Read the model definition and answer for the solid it produces. Units are mm, in the model's axes. Face numbers are marked on the shaded views. Coordinates: 2 decimals unless noted, no trailing zeros. Write each loop counter-clockwise with the first axis right and the second up, starting at its lowest first coordinate (ties: lowest second). Pieces come first, ordered by that corner, then holes. Notation, with made-up numbers: (66, -24) - (122, -24) arc R32 ccw to (122, 10) - close; hole circle Ø4 at (-12.75, 73.25). An arc over 180 degrees is marked (long way). Return JSON: item names as keys, results as strings.
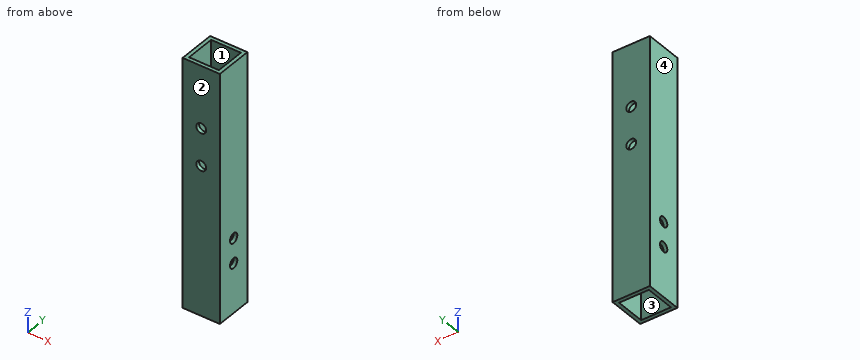
```python
from build123d import *

# Parameters (mm, degrees)
SKETCH_1_W          = 15
SKETCH_1_H          = 15
SKETCH_1_W_2        = 12
SKETCH_1_H_2        = 12
EXTRUDE_1_DEPTH     = 100
SKETCH_4_R          = 2
CUT_EXTRUDE_2_DEPTH = 75
SKETCH_5_R          = 2
CUT_EXTRUDE_3_DEPTH = 102.396498953


with BuildPart() as part:
    # 草图1 → 凸台-拉伸1 (new body)
    with BuildSketch(Plane.XY):
        Rectangle(SKETCH_1_W, SKETCH_1_H)
        Rectangle(SKETCH_1_W_2, SKETCH_1_H_2, mode=Mode.SUBTRACT)
    extrude(amount=EXTRUDE_1_DEPTH)

    # 草图4 → 切除-拉伸2 (cut)
    with BuildSketch(Plane.XZ.offset(7.5)):
        with Locations(Location((0, 75, 0), (0, 0, 270))):
            Circle(SKETCH_4_R)
        with Locations(Location((0, 60, 0), (0, 0, 270))):
            Circle(SKETCH_4_R)
    extrude(amount=-CUT_EXTRUDE_2_DEPTH, mode=Mode.SUBTRACT)

    # 草图5 → 切除-拉伸3 (cut, through all)
    with BuildSketch(Plane.ZY.offset(7.5)):
        with Locations((20, 0)):
            Circle(SKETCH_5_R)
        with Locations((30, 0)):
            Circle(SKETCH_5_R)
    extrude(amount=-CUT_EXTRUDE_3_DEPTH, mode=Mode.SUBTRACT)


solid = part.part
```
(1) A cutting plane is placed at D-D (x = -3.75). Determine the outline of the cut face in (y, z), and give its area (3 significant figures).
Answer:
{"outline": "(-7.5, 0) - (-6, 0) - (-6, 100) - (-7.5, 100) - close; (6, 0) - (7.5, 0) - (7.5, 100) - (6, 100) - close", "area": "300 mm²"}
(2) Straight lines are drawn through the part: line 1 (Y direction, x = 1, z = 38); line 2 (X direction, y = 7.15, z = 75). For each, find the intervals that lie inside material, in ascending order. Write a range as from..to.
Answer:
{"line 1": "-7.5..-6, 6..7.5", "line 2": "-7.5..-2, 2..7.5"}
(3) A cutting plane is placed at C-C (x = 0). Determine the outline of the cut face in (y, z).
Answer:
{"outline": "(-7.5, 0) - (-6, 0) - (-6, 58) - (-7.5, 58) - close; (-7.5, 62) - (-6, 62) - (-6, 73) - (-7.5, 73) - close; (-7.5, 77) - (-6, 77) - (-6, 100) - (-7.5, 100) - close; (6, 0) - (7.5, 0) - (7.5, 58) - (6, 58) - close; (6, 62) - (7.5, 62) - (7.5, 73) - (6, 73) - close; (6, 77) - (7.5, 77) - (7.5, 100) - (6, 100) - close"}
(4) A cutting plane is placed at A-A (z = 20). Determine the outline of the cut face in (x, y).
Answer:
{"outline": "(-7.5, -7.5) - (7.5, -7.5) - (7.5, -2) - (6, -2) - (6, -6) - (-6, -6) - (-6, -2) - (-7.5, -2) - close; (-7.5, 2) - (-6, 2) - (-6, 6) - (6, 6) - (6, 2) - (7.5, 2) - (7.5, 7.5) - (-7.5, 7.5) - close"}
(5) A cutting plane is placed at B-B (y = 0). Determine the outline of the cut face in (x, z), and give its area (3 significant figures).
Answer:
{"outline": "(-7.5, 0) - (-6, 0) - (-6, 18) - (-7.5, 18) - close; (-7.5, 22) - (-6, 22) - (-6, 28) - (-7.5, 28) - close; (-7.5, 32) - (-6, 32) - (-6, 100) - (-7.5, 100) - close; (6, 0) - (7.5, 0) - (7.5, 18) - (6, 18) - close; (6, 22) - (7.5, 22) - (7.5, 28) - (6, 28) - close; (6, 32) - (7.5, 32) - (7.5, 100) - (6, 100) - close", "area": "276 mm²"}
(6) Determine the mould class of the marked faces 1, 2, 3 and 4 for opening direction X: +X half, -X half, draft (parallel to the pull), parting line (faces both ways), or undercut.
Answer:
{"face 1": "undercut", "face 2": "draft", "face 3": "undercut", "face 4": "-X half"}
